from build123d import *

# Parameters (mm, degrees)
SKETCH1_W                                        = 30
SKETCH1_H                                        = 57
BOSS_EXTRUDE1_DEPTH                              = 4
SKETCH2_R                                        = 5
CUT_EXTRUDE1_DEPTH                               = 65.536811201
F_4_0_4_DIAMETER_HOLE1_D                         = 4
SKETCH12_W                                       = 14.5
SKETCH12_H                                       = 24
CUT_EXTRUDE2_DEPTH                               = 65.536811201
SKETCH13_W                                       = 42.673617324
SKETCH13_H                                       = 65.779819875
CUT_EXTRUDE5_DEPTH                               = 4
F_4_0_4_DIAMETER_HOLE6_D                         = 4
CBORE_FOR_M3_PAN_HEAD_MACHINE_SCREW7_D           = 3.2
CBORE_FOR_M3_PAN_HEAD_MACHINE_SCREW7_CBORE_D     = 9
CBORE_FOR_M3_PAN_HEAD_MACHINE_SCREW7_CBORE_DEPTH = 1
CSK_FOR_M3_FLAT_HEAD_MACHINE_SCREW1_D            = 3.2
CSK_FOR_M3_FLAT_HEAD_MACHINE_SCREW1_CSINK_D      = 4
CSK_FOR_M3_FLAT_HEAD_MACHINE_SCREW1_CSINK_ANGLE  = 90
CUT_EXTRUDE6_DEPTH                               = 65.536811201
CUT_EXTRUDE6_DEPTH_BACK                          = 65.536811201
SKETCH45_W                                       = 4
SKETCH45_H                                       = 33
SKETCH46_W                                       = 0.1
SKETCH46_H                                       = 57
CUT_EXTRUDE7_DEPTH                               = 63.777384463


with BuildPart() as part:
    # Sketch1 → Boss-Extrude1 (new body)
    with BuildSketch(Plane(origin=(0, 0, 0), x_dir=(0, 0, -1), z_dir=(1, 0, 0))):
        with Locations((-15, 28.5)):
            Rectangle(SKETCH1_W, SKETCH1_H)
    boss_extrude1 = extrude(amount=-BOSS_EXTRUDE1_DEPTH)

    # Sketch2 → Cut-Extrude1 (cut, through all)
    with BuildSketch(Plane(origin=(0, 0, 0), x_dir=(0, 0, -1), z_dir=(1, 0, 0))):
        with Locations((-7, 23.5)):
            Circle(SKETCH2_R)
    cut_extrude1 = extrude(amount=-CUT_EXTRUDE1_DEPTH, mode=Mode.SUBTRACT)

    # Ø4.0 (4) Diameter Hole1 (through all)
    with Locations(Plane(origin=(0, 4.5, 7), x_dir=(0, 0, 1), z_dir=(1, 0, 0))):
        with Locations((0, 0)):
            Hole(F_4_0_4_DIAMETER_HOLE1_D / 2)

    # Sketch12 → Cut-Extrude2 (cut, through all)
    with BuildSketch(Plane(origin=(0, 0, 0), x_dir=(0, 0, -1), z_dir=(1, 0, 0))):
        with Locations((-22.75, 12)):
            Rectangle(SKETCH12_W, SKETCH12_H)
    cut_extrude2 = extrude(amount=-CUT_EXTRUDE2_DEPTH, mode=Mode.SUBTRACT)

    # Mirror7: Boss-Extrude1, Cut-Extrude1, Cut-Extrude2 across plane
    add(boss_extrude1.mirror(Plane(origin=(0, 0, 0), x_dir=(0, 0, 1), z_dir=(1, 0, 0))))
    add(cut_extrude1.mirror(Plane(origin=(0, 0, 0), x_dir=(0, 0, 1), z_dir=(1, 0, 0))), mode=Mode.SUBTRACT)
    add(cut_extrude2.mirror(Plane(origin=(0, 0, 0), x_dir=(0, 0, 1), z_dir=(1, 0, 0))), mode=Mode.SUBTRACT)

    # Sketch13 → Cut-Extrude5 (cut)
    with BuildSketch(Plane.ZY.offset(4)):
        with Locations((15.520409967, 28.395918007)):
            Rectangle(SKETCH13_W, SKETCH13_H)
    extrude(amount=-CUT_EXTRUDE5_DEPTH, mode=Mode.SUBTRACT)

    # Ø4.0 (4) Diameter Hole6 (through all)
    with Locations(Plane(origin=(0, 4.5, 7), x_dir=(0, 0, -1), z_dir=(-1, 0, 0))):
        with Locations((0, 0)):
            Hole(F_4_0_4_DIAMETER_HOLE6_D / 2)

    # CBORE for M3 Pan Head Machine Screw7 (through all)
    with Locations(Plane(origin=(4, 41.360571099, 16), x_dir=(0, 0, 1), z_dir=(1, 0, 0))):
        with Locations((0, 0)):
            CounterBoreHole(CBORE_FOR_M3_PAN_HEAD_MACHINE_SCREW7_D / 2, CBORE_FOR_M3_PAN_HEAD_MACHINE_SCREW7_CBORE_D / 2, CBORE_FOR_M3_PAN_HEAD_MACHINE_SCREW7_CBORE_DEPTH)

    # CSK for M3 Flat Head Machine Screw1 (through all)
    with Locations(Plane(origin=(0, 30.032608687, 19.33966579), x_dir=(0, 0, -1), z_dir=(-1, 0, 0))):
        with Locations((0, 0), (14.431341448, -7.272)):
            CounterSinkHole(CSK_FOR_M3_FLAT_HEAD_MACHINE_SCREW1_D / 2, CSK_FOR_M3_FLAT_HEAD_MACHINE_SCREW1_CSINK_D / 2, counter_sink_angle=CSK_FOR_M3_FLAT_HEAD_MACHINE_SCREW1_CSINK_ANGLE)

    # Sketch45 → Cut-Extrude6 (cut, two sides: drawn at the far end of the back side and taken through both)
    with BuildSketch(Plane(origin=(4, 0, 0), x_dir=(0, 0, -1), z_dir=(1, 0, 0)).offset(-CUT_EXTRUDE6_DEPTH_BACK)):
        with Locations((-28, 40.5)):
            Rectangle(SKETCH45_W, SKETCH45_H)
    extrude(amount=CUT_EXTRUDE6_DEPTH + CUT_EXTRUDE6_DEPTH_BACK, mode=Mode.SUBTRACT)

    # Sketch46 → Cut-Extrude7 (cut, through all)
    with BuildSketch(Plane(origin=(0, 0, 0), x_dir=(-1, 0, 0), z_dir=(0, 0, -1))):
        with Locations((-3.95, 28.5)):
            Rectangle(SKETCH46_W, SKETCH46_H)
    extrude(amount=-CUT_EXTRUDE7_DEPTH, mode=Mode.SUBTRACT)


solid = part.part
Check sheet for the modelled part. Datum: model origin and axes. Units: mm. A direction names the side the tool comes from. Round coordinates to 2 decimals unless told otherwise and drop trailing zeros. Loops run counter-clockwise (first coordinate to the right, second up) from the corner with the lowest first, then second, coordinate; pieces in that order, holes last. Notation, with made-up numbers: (18.5, 75) -> (71.5, 75) arc R18 ccw to (71.5, 81) -> close; hole circle Ø3 at (28.25, -11). An arc over 180 degrees is marked (long way). Put each result on its own line as item: value. Start each with the question number.
1. Section check B-B (z = 10.25). Enter the section's corners in (x, y).
2. Access from +Z, -Z, +X, -X, +Y, -Y to the whole of each face (thin tool, end or side, straight path). Record for faces 4 (the face through (2, 40, 26)), 5 (the face through (3.456, 45.754, 15.024)).
3. Section check C-C (x = 2.1). Enter the section's corners in (y, z), plus the area to 3 significant figures.
4. Draft check along Y on faces 1 (the face through (2, 24, 21)), 2 (the face through (2, 12, 15.5)), 3 (the face through (1.977, 19.064, 4.693)). Enter one of: +Y half, -Y half, draft (parallel to the pull), parting line (faces both ways), or undercut.
5. Scan lines: probe 1 along Y at (x, z) = (2.8, 7); probe 2 along Y at (x, z) = (0.8, 20); probe 3 along Y at (x, z) = (0.95, 2.75). Record each from-to range of solid material in increasing order.
6. Gauge pin test, flat end, axial feed: pin 1 (6 mm diameter, centred on y = 23.5, z = 7, fed in from -X). Record the tip position at first contact, or that the pin passes through.
7. Section check A-A (y = 4.5). Enter the section's corners in (x, z).
Findings:
1. outline: (0, 0) -> (3.9, 0) -> (3.9, 19.7) -> (0, 19.7) -> close; (0, 27.3) -> (3.9, 27.3) -> (3.9, 57) -> (0, 57) -> close
2. face 4: +Z, +X, -X, +Y, -Y
2. face 5: +X
3. outline: (0, 0) -> (57, 0) -> (57, 26) -> (24, 26) -> (24, 15.5) -> (0, 15.5) -> close; hole circle Ø4 at (4.5, 7); hole circle Ø10 at (23.5, 7); hole circle Ø3.2 at (30.03, 19.34); hole circle Ø3.2 at (37.3, 4.91); hole circle Ø3.2 at (41.36, 16)
3. area: 1,110 mm^2
4. face 1: -Y half
4. face 2: draft
4. face 3: undercut
5. probe 1: y = 0 to 2.5, 6.5 to 18.5, 28.5 to 57
5. probe 2: y = 24 to 28.58, 31.49 to 57
5. probe 3: y = 0 to 20.87, 26.13 to 57
6. pin 1: passes through
7. outline: (0, 0) -> (3.9, 0) -> (3.9, 5) -> (0, 5) -> close; (0, 9) -> (3.9, 9) -> (3.9, 15.5) -> (0, 15.5) -> close
